from build123d import *

# Parameters (mm, degrees)
SKETCH1_R           = 3.25
SKETCH1_R_2         = 1.9
BOSS_EXTRUDE1_DEPTH = 5


with BuildPart() as part:
    # Sketch1 → Boss-Extrude1 (new body)
    with BuildSketch(Plane.XY):
        with BuildLine():
            Line((-295, -10), (5, -10))
            ThreePointArc((5, -10), (8.535533906, -8.535533906), (10, -5))
            Line((10, -5), (10, 245))
            ThreePointArc((10, 245), (8.535533906, 248.535533906), (5, 250))
            Line((5, 250), (-295, 250))
            ThreePointArc((-295, 250), (-298.535533906, 248.535533906), (-300, 245))
            Line((-300, 245), (-300, -5))
            ThreePointArc((-300, -5), (-298.535533906, -8.535533906), (-295, -10))
        make_face()
        Circle(SKETCH1_R, mode=Mode.SUBTRACT)
        with Locations((0, 240)):
            Circle(SKETCH1_R, mode=Mode.SUBTRACT)
        with Locations((-290, 239)):
            Circle(SKETCH1_R, mode=Mode.SUBTRACT)
        with Locations((-290, 1)):
            Circle(SKETCH1_R, mode=Mode.SUBTRACT)
        with Locations(Location((-286.899999971, 51.217380491, 0), (0, 0, 180))):
            Circle(SKETCH1_R_2, mode=Mode.SUBTRACT)
        with Locations(Location((-286.899999971, 17.782619509, 0), (0, 0, 180))):
            Circle(SKETCH1_R_2, mode=Mode.SUBTRACT)
        with Locations((-3.100000029, 17.782619509)):
            Circle(SKETCH1_R_2, mode=Mode.SUBTRACT)
        with Locations((-3.100000029, 51.217380491)):
            Circle(SKETCH1_R_2, mode=Mode.SUBTRACT)
    extrude(amount=BOSS_EXTRUDE1_DEPTH)


solid = part.part
CAD build for the part. Positions are in the model's coordinates, mm. Round coordinates to 2 decimals unless told otherwise and drop trailing zeros. Answer as a JSON object with one key per item and string values.
(1) Pin check, flat tips, straight feed: P1, Ø10.5, axis at x = 0, y = 0, coming from the +Z side; P2, Ø2.5, axis at x = -3.1, y = 17.78, coming from the +Z side. Stop position of each tip, or through.
Reported:
{"P1": "stops at z = 5", "P2": "passes through"}
(2) Probe probe 1 along Y at (x, z) = (0, 1.15); probe 2 along X at (y, z) = (239, 3.95); probe 3 along Y at (x, z) = (-290, 3.5). List the from-to ranges inside material, lowest first. Write a range as [from, to].
Reported:
{"probe 1": "y = [-10, -3.25], [3.25, 236.75], [243.25, 250]", "probe 2": "x = [-300, -293.25], [-286.75, -3.09], [3.09, 10]", "probe 3": "y = [-10, -2.25], [4.25, 235.75], [242.25, 250]"}
(3) Two-plate mould, pull along X, no slides. Class faces 1 (the face through (-147, 122, 0)), 2 (the face through (1.75, 242.74, 2.46)): +X half, -X half, draft (parallel to the pull), parting line (faces both ways), or undercut.
Reported:
{"face 1": "draft", "face 2": "undercut"}
